The drawing under review shows one solid part. Ordinate dimensions are in mm from its lowest x, y, z. Coordinates: 2 decimals unless noted, no trailing zeros. Loops run counter-clockwise (first coordinate to the right, second up) from the corner with the lowest first, then second, coordinate; pieces in that order, holes last. Notation, with made-up numbers: M 88.5,59.25 L 137.5,59.25 A32 ccw 137.5,90.25 Z; hole C 81,84 d4. An arc over 180 degrees is marked long. Put each result on its own line as item: value.
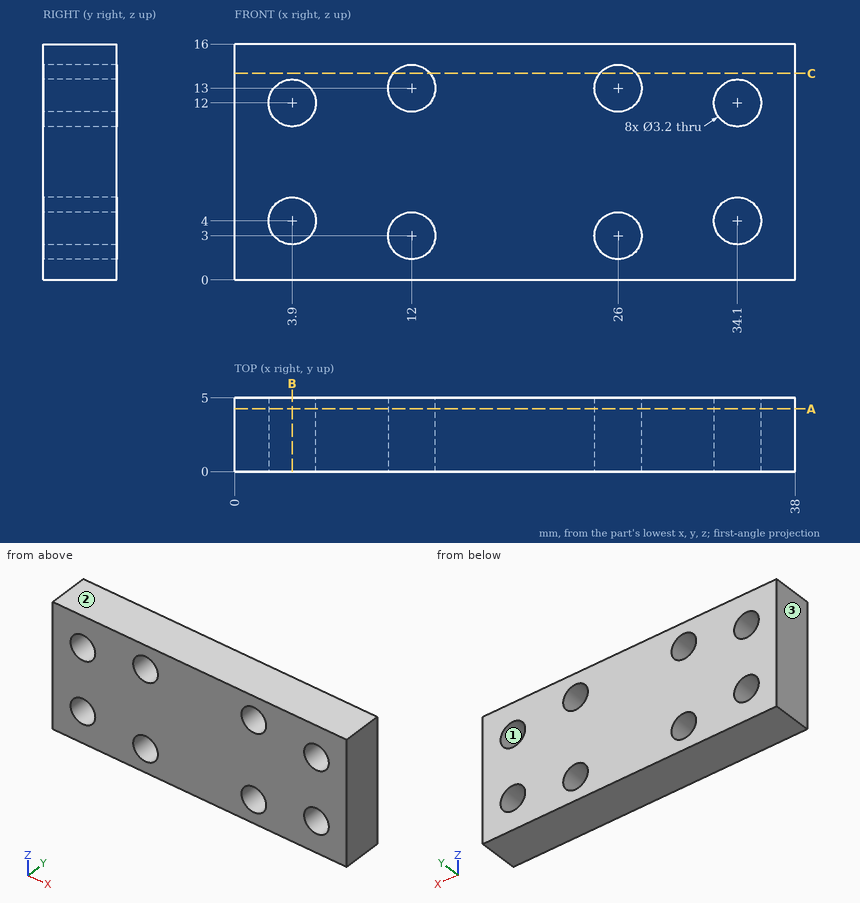
(1) Add section A-A (y = 4.25). State how many separate pieces and enclosed holes the cut face has, plus the area to 3 significant figures.
Determined:
separate pieces: 1
enclosed holes: 8
area: 544 mm^2
(2) For pin 1 (3 mm diameter, centred on x = 34.1, z = 4, fed in from -Y), flat-tipped, find the tip position at first contact; note if it passes through.
Determined:
pin 1: passes through
(3) Wall thickness on line 1 along Z through (x, y) = (3.9, 3.9); line 2 along Z through (x, y) = (12, 4); line 3 along X through (y, z) = (4.5, 14): over which ranges is each line inside the solid? List them lowest first. Write a range as [from, to].
Determined:
line 1: z = [0, 2.4], [5.6, 10.4], [13.6, 16]
line 2: z = [0, 1.4], [4.6, 11.4], [14.6, 16]
line 3: x = [0, 10.75], [13.25, 24.75], [27.25, 38]
(4) Add section C-C (z = 14). Write out the cut boundary in (x, y).
Determined:
outline: M 0,0 L 10.75,0 L 10.75,5 L 0,5 Z; M 13.25,0 L 24.75,0 L 24.75,5 L 13.25,5 Z; M 27.25,0 L 38,0 L 38,5 L 27.25,5 Z
(5) Add section B-B (x = 3.9). Write out the cut boundary in (y, z).
Determined:
outline: M 0,0 L 5,0 L 5,2.4 L 0,2.4 Z; M 0,5.6 L 5,5.6 L 5,10.4 L 0,10.4 Z; M 0,13.6 L 5,13.6 L 5,16 L 0,16 Z
(6) Draft analysis for pull direction X (two halves, no side actions). For the marked faces 1, 2 and 3, state which applies: +X half, -X half, draft (parallel to the pull), parting line (faces both ways), or undercut.
Determined:
face 1: undercut
face 2: draft
face 3: -X half
